Part print with two shaded views. Sizes in mm from the minimum x, y, z corner. A direction names the side the tool comes from. Round coordinates to 2 decimals unless told otherwise and drop trailing zeros. Loops run counter-clockwise (first coordinate to the right, second up) from the corner with the lowest first, then second, coordinate; pieces in that order, holes last. Notation, with made-up numbers: (24.5, 5) -> (58.5, 5) arc R19 ccw to (58.5, 36) -> close; hole circle Ø8 at (70, -37). An arc over 180 degrees is marked (long way). Use a Markdown table: item, result. Add a question column.
Item 1: Probe line 1 (Y direction, x = 6, z = 7.75); line 2 (Z direction, x = 3.25, y = 6.5); line 3 (Z direction, x = 0.5, y = 13). List the from-to ranges inside material, lowest first. Write a range as [from, to].
Item 2: Two-plate mould, pull along X, no slides. Class the marked faces 4, 5, 6 and 7: pulls with the +X half, pulls with the -X half, needs draft (parallel to the pull), parting line crosses it, or undercut.
Item 3: Flat gauge pins, fed straight in: pin 1 (2 mm diameter, centred on y = 7, z = 2, fed in from +X); pin 2 (3.5 mm diameter, centred on x = 9, y = 7.5, fed in from +Z). Where does each tip first touch, or does it go through?
Item 4: Cut at B-B, the plane y = 12.5. List the corners of the cut face in (x, z), plus the area to 3 significant figures.
Item 5: Which spindle directions (+Z, -Z, +X, -X, +Y, -Y) get a long thin tool onto all of the face, cutting with end or side? Do the marked faces 1, 2 and 3. Say none if no direction does.
Item 6: Cut at D-D, the plane y = 11. List the corners of the cut face in (x, z).
Item 7: Cut at C-C, the plane x = 2.5. List the corners of the cut face in (y, z).
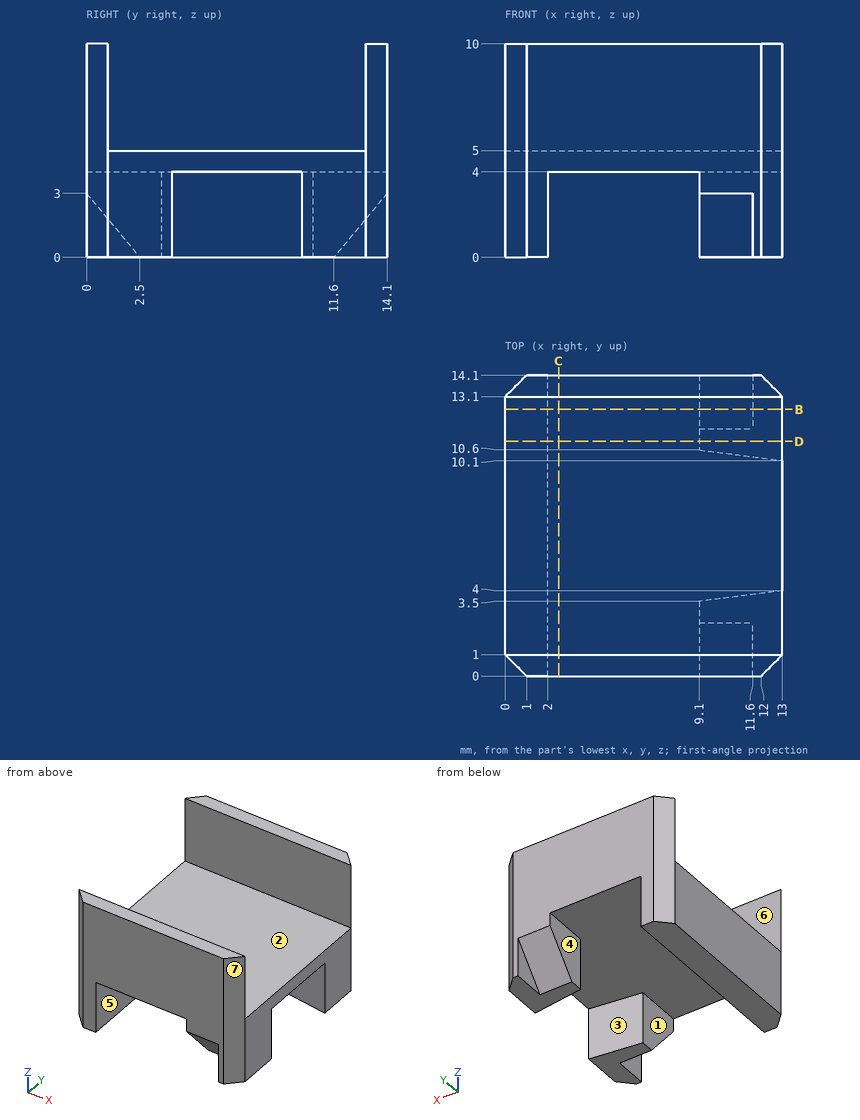
A:
| question | item | result |
|---|---|---|
| 1 | line 1 | y = [0, 1], [13.1, 14.1] |
| 1 | line 2 | z = [4, 5] |
| 1 | line 3 | z = [0, 5] |
| 2 | face 4 | undercut |
| 2 | face 5 | undercut |
| 2 | face 6 | needs draft |
| 2 | face 7 | pulls with the +X half |
| 3 | pin 1 | stops at x = 2 |
| 3 | pin 2 | stops at z = 5 |
| 4 | outline | (0, 0) -> (2, 0) -> (2, 4) -> (9.1, 4) -> (9.1, 1.08) -> (11.6, 1.08) -> (11.6, 0) -> (13, 0) -> (13, 5) -> (0, 5) -> close |
| 4 | area | 33.9 mm^2 |
| 5 | face 1 | -Z, +Y, -Y |
| 5 | face 2 | +Z, +X, -X |
| 5 | face 3 | -Z |
| 6 | outline | (0, 0) -> (2, 0) -> (2, 4) -> (9.1, 4) -> (9.1, 0) -> (13, 0) -> (13, 5) -> (0, 5) -> close |
| 7 | outline | (0, 4) -> (14.1, 4) -> (14.1, 10) -> (13.1, 10) -> (13.1, 5) -> (1, 5) -> (1, 10) -> (0, 10) -> close |
